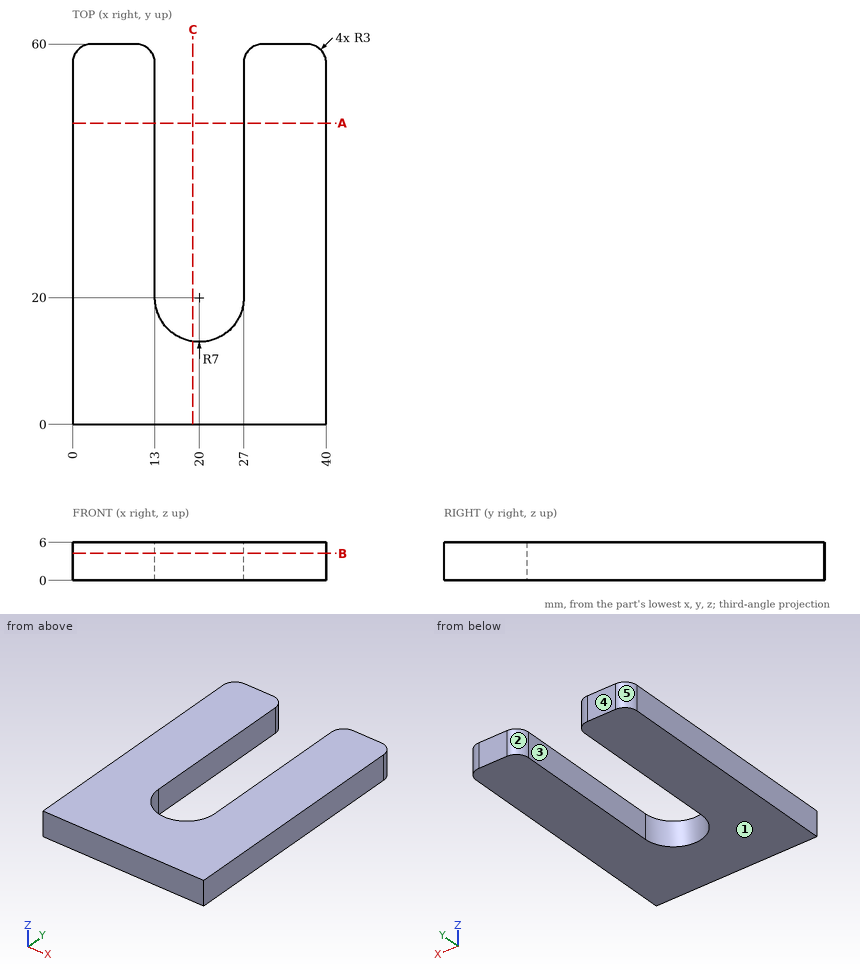
The drawing under review shows one solid part. Ordinate dimensions are in mm from its lowest x, y, z. A direction names the side the tool comes from. Give positions to 0.01 mm unless a question says otherwise; leave off trailing zeros. Write each loop counter-clockwise with the first axis right and the second up, starting at its lowest first coordinate (ties: lowest second). Pieces come first, ordered by that corner, then holes. Notation, with made-up numbers: (64, 66) - (120, 66) arc R16 cw to (120, 82) - close; hole circle Ø7 at (-28.5, 10.5). An arc over 180 degrees is marked (long way). Answer in a Markdown table with one row per item. Add a question column.
1. Draft analysis for pull direction X (two halves, no side actions). For the marked faces 3, 4 and 5, state which applies: +X half, -X half, draft (parallel to the pull), parting line (faces both ways), or undercut.
2. We need section A-A on y = 47.5. Write out the cut boundary in (x, z), then the cut area to 3 significant figures.
3. Wall thickness on line 1 along X through (y, z) = (23.5, 3.9); line 2 along X through (y, z) = (19, 4.5); line 3 along Y through (x, z) = (28.5, 0.45): over which ranges is each line inside the solid? List them lowest first. Write a range as [from, to].
4. We need section B-B on z = 4.25. Write out the cut boundary in (x, y).
5. Tool access review of the marked faces 1 and 2: name each direction out of +Z, -Z, +X, -X, +Y, -Y from which nothing blocks a thin tool from reaching the whole face with its end or side.
6. We need section C-C on x = 19. Write out the cut boundary in (y, z).
Ans:
| question | item | result |
|---|---|---|
| 1 | face 3 | undercut |
| 1 | face 4 | draft |
| 1 | face 5 | -X half |
| 2 | outline | (0, 0) - (13, 0) - (13, 6) - (0, 6) - close; (27, 0) - (40, 0) - (40, 6) - (27, 6) - close |
| 2 | area | 156 mm^2 |
| 3 | line 1 | x = [0, 13], [27, 40] |
| 3 | line 2 | x = [0, 13.07], [26.93, 40] |
| 3 | line 3 | y = [0, 59.6] |
| 4 | outline | (0, 0) - (40, 0) - (40, 57) arc R3 ccw to (37, 60) - (30, 60) arc R3 ccw to (27, 57) - (27, 20) arc R7 cw to (13, 20) - (13, 57) arc R3 ccw to (10, 60) - (3, 60) arc R3 ccw to (0, 57) - close |
| 5 | face 1 | -Z, +X, -X, +Y, -Y |
| 5 | face 2 | +Z, -Z, +Y |
| 6 | outline | (0, 0) - (13.07, 0) - (13.07, 6) - (0, 6) - close |
